CAD build for the part. Positions are in the model's coordinates, mm. Face numbers are marked on the shaded views. A direction names the side the tool comes from. Give positions to 0.01 mm unless a question says otherwise; leave off trailing zeros. Loops run counter-clockwise (first coordinate to the right, second up) from the corner with the lowest first, then second, coordinate; pieces in that order, holes last. Notation, with made-up numbers: M 56,14.25 L 76,14.25 A32 ccw 76,48.25 Z; hole C 42.25,82 d7. An arc over 180 degrees is marked long. Answer as CSV lines item,"result".
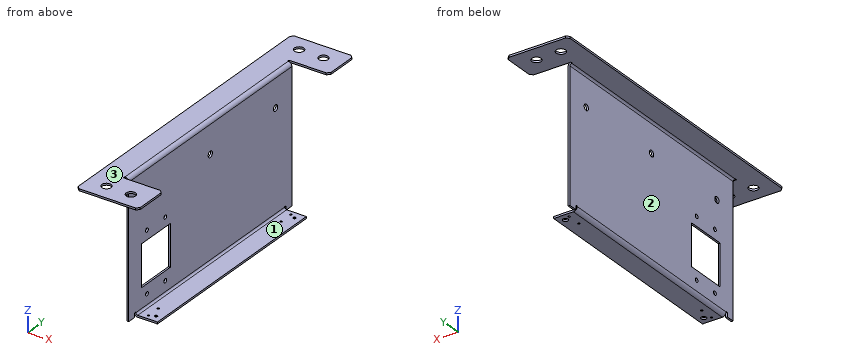
from build123d import *

# Parameters (mm, degrees)
SKETCH_1_R          = 5
EXTRUDE_1_DEPTH     = 2
SKETCH_2_W          = 2
SKETCH_2_H          = 250
EXTRUDE_2_DEPTH     = 144
SKETCH_3_W          = 2
SKETCH_3_H          = 228
EXTRUDE_3_DEPTH     = 23
SKETCH_4_W          = 4.5
SKETCH_4_H          = 2
CUT_EXTRUDE_1_DEPTH = 2
SKETCH_5_W          = 4.5
SKETCH_5_H          = 2
CUT_EXTRUDE_2_DEPTH = 2
FILLET_3_R          = 2
FILLET_4_R          = 4
SKETCH_6_R          = 1.1
SKETCH_6_R_2        = 1.5
CUT_EXTRUDE_3_DEPTH = 2
CHAMFER_1_SIZE      = 1.3
SKETCH_8_R          = 3.25
SKETCH_8_R_2        = 2.1
SKETCH_8_W          = 44
SKETCH_8_H          = 44
CUT_EXTRUDE_4_DEPTH = 2


with BuildPart() as part:
    # Эскиз1 → Вытянуть1 (new body)
    with BuildSketch(Plane.XY):
        Polygon((-15.389384289, -165), (44.610615711, -165), (47.610615711, -162), (47.610615711, -130), (44.610615711, -127), (9.610615711, -127), (9.610615711, 127), (44.610615711, 127), (47.610615711, 130), (47.610615711, 162), (44.610615711, 165), (-15.389384289, 165), (-18.389384289, 162), (-18.389384289, -162), align=None)
        with Locations((1.610615711, -147.5)):
            Circle(SKETCH_1_R, mode=Mode.SUBTRACT)
        with Locations((27.610615711, -147.5)):
            Circle(SKETCH_1_R, mode=Mode.SUBTRACT)
        with Locations(Location((27.610615711, 147.5, 0), (0, 0, 180))):
            Circle(SKETCH_1_R, mode=Mode.SUBTRACT)
        with Locations(Location((1.610615711, 147.5, 0), (0, 0, 180))):
            Circle(SKETCH_1_R, mode=Mode.SUBTRACT)
    extrude(amount=EXTRUDE_1_DEPTH)

    # Эскиз2 → Вытянуть2 (add)
    with BuildSketch(Plane.XY.offset(2)):
        with Locations((8.610615711, 0)):
            Rectangle(SKETCH_2_W, SKETCH_2_H)
    extrude(amount=-EXTRUDE_2_DEPTH)

    # Эскиз3 → Вытянуть3 (add)
    with BuildSketch(Plane(origin=(9.610615711, 0, 0), x_dir=(0, 0, -1), z_dir=(1, 0, 0))):
        with Locations((141, 0)):
            Rectangle(SKETCH_3_W, SKETCH_3_H)
    extrude(amount=EXTRUDE_3_DEPTH)

    # Эскиз4 → Вырез-Вытянуть1 (cut)
    with BuildSketch(Plane.XY.offset(2)):
        with Locations((7.360615711, 126)):
            Rectangle(SKETCH_4_W, SKETCH_4_H)
        with Locations((7.360615711, -126)):
            Rectangle(SKETCH_4_W, SKETCH_4_H)
    extrude(amount=-CUT_EXTRUDE_1_DEPTH, mode=Mode.SUBTRACT)

    # Эскиз5 → Вырез-Вытянуть2 (cut)
    with BuildSketch(Plane(origin=(9.610615711, 0, 0), x_dir=(0, 0, -1), z_dir=(1, 0, 0))):
        with Locations((139.75, -115)):
            Rectangle(SKETCH_5_W, SKETCH_5_H)
        with Locations((139.75, 115)):
            Rectangle(SKETCH_5_W, SKETCH_5_H)
    extrude(amount=-CUT_EXTRUDE_2_DEPTH, mode=Mode.SUBTRACT)

    # Скругление3
    fillet_3_edges = [part.edges().sort_by_distance(p)[0] for p in [
        (9.610615711, 0, -140),
        (7.610615711, 0, 0),
    ]]
    fillet(fillet_3_edges, radius=FILLET_3_R)

    # Скругление4
    fillet_4_edges = [part.edges().sort_by_distance(p)[0] for p in [
        (7.610615711, 0, -142),
        (9.610615711, 0, 2),
    ]]
    fillet(fillet_4_edges, radius=FILLET_4_R)

    # Эскиз6 → Вырез-Вытянуть3 (cut)
    with BuildSketch(Plane(origin=(0, 0, -142), x_dir=(-1, 0, 0), z_dir=(0, 0, -1))):
        with Locations(Location((-19.610615711, -94, 0), (0, 0, 180))):
            Circle(SKETCH_6_R)
        with Locations((-25.610615711, -106)):
            Circle(SKETCH_6_R_2)
        with Locations((-25.610615711, 106)):
            Circle(SKETCH_6_R_2)
        with Locations(Location((-19.610615711, -109, 0), (0, 0, 180))):
            Circle(SKETCH_6_R)
        with Locations((-19.610615711, 109)):
            Circle(SKETCH_6_R)
        with Locations((-19.610615711, 94)):
            Circle(SKETCH_6_R)
    extrude(amount=-CUT_EXTRUDE_3_DEPTH, mode=Mode.SUBTRACT)

    # Фаска1
    chamfer_1_edges = [part.edges().sort_by_distance(p)[0] for p in [
        (27.110615711, -106, -142),
        (27.110615711, 106, -142),
    ]]
    chamfer(chamfer_1_edges, length=CHAMFER_1_SIZE)

    # Эскиз8 → Вырез-Вытянуть4 (cut)
    with BuildSketch(Plane(origin=(9.610615711, 0, 0), x_dir=(0, 0, -1), z_dir=(1, 0, 0))):
        with Locations((32, 0)):
            Circle(SKETCH_8_R)
        with Locations((32, -100)):
            Circle(SKETCH_8_R)
        with Locations(Location((32, 100, 0), (0, 0, 180))):
            Circle(SKETCH_8_R)
        with Locations((63, -97)):
            Circle(SKETCH_8_R_2)
        with Locations((127, -97)):
            Circle(SKETCH_8_R_2)
        with Locations((127, -69)):
            Circle(SKETCH_8_R_2)
        with Locations((63, -69)):
            Circle(SKETCH_8_R_2)
        with Locations((95, -83)):
            Rectangle(SKETCH_8_W, SKETCH_8_H)
    extrude(amount=-CUT_EXTRUDE_4_DEPTH, mode=Mode.SUBTRACT)


solid = part.part
1) Band-saw the part on C-C on z = -32. Give the cut face in (x, y).
Answer below:
outline,"M 7.61,-125 L 9.61,-125 L 9.61,-103.25 L 7.61,-103.25 Z; M 7.61,-96.75 L 9.61,-96.75 L 9.61,-3.25 L 7.61,-3.25 Z; M 7.61,3.25 L 9.61,3.25 L 9.61,96.75 L 7.61,96.75 Z; M 7.61,103.25 L 9.61,103.25 L 9.61,125 L 7.61,125 Z"
2) Drill centre lines: line 1 (Y direction, x = 8.1, z = -32); line 2 (Y direction, x = 9, z = -127); line 3 (X direction, y = -21, z = -96). Where is each one in solid material? Low to high. Write a range as from..to.
Answer below:
line 1,"y = -125..-103.25, -96.75..-3.25, 3.25..96.75, 103.25..125"
line 2,"y = -125..-99.1, -94.9..-71.1, -66.9..125"
line 3,"x = 7.61..9.61"
3) Band-saw the part on B-B on y = -147.5. Give the cut face in (x, z).
Answer below:
outline,"M -18.39,0 L -3.39,0 L -3.39,2 L -18.39,2 Z; M 6.61,0 L 22.61,0 L 22.61,2 L 6.61,2 Z; M 32.61,0 L 47.61,0 L 47.61,2 L 32.61,2 Z"
4) Flat gauge pins, fed straight in: pin 1 (2.5 mm diameter, centred on x = 8, z = -51.5, fed in from -Y); pin 2 (5 mm diameter, centred on y = -110, z = -93.5, fed in from -X); pin 3 (2.5 mm diameter, centred on y = -97, z = -127, fed in from +X); pin 4 (1 mm diameter, centred on y = 126, z = 1, fed in from +X). Where does each tip first touch, or does it go through?
Answer below:
pin 1,"stops at y = -125"
pin 2,"stops at x = 7.61"
pin 3,"passes through"
pin 4,"stops at x = 5.11"
5) Which spindle directions (+Z, -Z, +X, -X, +Y, -Y) get a long thin tool onto all of the face, cutting with end or side? Do the marked faces 1, 2 and 3. Say none if no direction does.
Answer below:
face 1,"+Z, +X, +Y, -Y"
face 2,"-Z, -X, +Y, -Y"
face 3,"+Z, +X, -X, +Y, -Y"
6) Band-saw the part on D-D on y = 0. Give the cut face in (x, z), and give its area (3 significant figures).
Answer below:
outline,"M -18.39,0 L 5.61,0 A2 cw 7.61,-2 L 7.61,-28.75 L 9.61,-28.75 L 9.61,-2 A4 ccw 5.61,2 L -18.39,2 Z; M 7.61,-138 A4 ccw 11.61,-142 L 32.61,-142 L 32.61,-140 L 11.61,-140 A2 cw 9.61,-138 L 9.61,-35.25 L 7.61,-35.25 Z"
area,"368 mm^2"
7) Band-saw the part on A-A on z = -83. Give the cut face in (x, y), and give its area (3 significant figures).
Answer below:
outline,"M 7.61,-125 L 9.61,-125 L 9.61,-105 L 7.61,-105 Z; M 7.61,-61 L 9.61,-61 L 9.61,125 L 7.61,125 Z"
area,"412 mm^2"
